Check sheet for the modelled part. Datum: model origin and axes. Units: mm. A direction names the side the tool comes from. Give positions to 0.01 mm unless a question says otherwise; leave off trailing zeros. Write each loop counter-clockwise with the first axis right and the second up, starting at its lowest first coordinate (ties: lowest second). Pieces come first, ordered by that corner, then holes.
from build123d import *

# Parameters (mm, degrees)
SKETCH1_W           = 90
SKETCH1_H           = 45
BOSS_EXTRUDE1_DEPTH = 117
SKETCH1_3_W         = 90
SKETCH1_3_H         = 36
BOSS_EXTRUDE2_DEPTH = 45
BOSS_EXTRUDE3_DEPTH = 27
RIB2_REACH          = 188.435
SKETCH2_WALL_W      = 425.781638764
SKETCH2_WALL_H      = 18
CUT_EXTRUDE1_REACH  = 158.087
SKETCH3_R           = 27


with BuildPart() as part:
    # Sketch1 → Boss-Extrude1 (new body)
    with BuildSketch(Plane.XY):
        with Locations((0, 22.5)):
            Rectangle(SKETCH1_W, SKETCH1_H)
    extrude(amount=BOSS_EXTRUDE1_DEPTH)

    # Sketch1_3 → Boss-Extrude2 (add)
    with BuildSketch(Plane.XY):
        with Locations((0, 63)):
            Rectangle(SKETCH1_3_W, SKETCH1_3_H)
    extrude(amount=BOSS_EXTRUDE2_DEPTH)

    # Sketch1_4 → Boss-Extrude3 (add)
    with BuildSketch(Plane.XY):
        with BuildLine():
            ThreePointArc((-45, 93), (0, 138), (45, 93))
            Line((45, 93), (45, 81))
            Line((45, 81), (-45, 81))
            Line((-45, 81), (-45, 93))
        make_face()
        with BuildLine():
            Line((-27, 93), (27, 93))
            ThreePointArc((27, 93), (0, 120), (-27, 93))
        make_face(mode=Mode.SUBTRACT)
    extrude(amount=BOSS_EXTRUDE3_DEPTH)

    # Sketch2 wall → Rib2 (add, up to next)
    with BuildSketch(Plane(origin=(0, 63, 63), x_dir=(0, -0.707106781187, 0.707106781187), z_dir=(0, -0.707106781187, -0.707106781187)), mode=Mode.PRIVATE) as rib2_sk1:
        Rectangle(SKETCH2_WALL_W, SKETCH2_WALL_H)
    rib2_tool1 = extrude(rib2_sk1.sketch, amount=RIB2_REACH, mode=Mode.PRIVATE) - part.part
    add(rib2_tool1.solids().sort_by_distance((0, 63, 63))[0])

    # Sketch3 → Cut-Extrude1 (cut, up to next)
    with BuildSketch(Plane(origin=(0, 45, 0), x_dir=(1, 0, 0), z_dir=(0, 1, 0)), mode=Mode.PRIVATE) as cut_extrude1_sk1:
        with Locations((0, -117)):
            Circle(SKETCH3_R)
    cut_extrude1_tool1 = extrude(cut_extrude1_sk1.sketch, amount=-CUT_EXTRUDE1_REACH, mode=Mode.PRIVATE) & part.part
    add(cut_extrude1_tool1.solids().sort_by_distance((0, 45, 117))[0], mode=Mode.SUBTRACT)


solid = part.part
1) Gauge pin test, flat ends, axial feed: pin 1 (5 mm diameter, centred on x = -28, y = 99.5, fed in from +Z); pin 2 (11 mm diameter, centred on x = -20, y = 70, fed in from +Z); pin 3 (11 mm diameter, centred on y = 59, z = 71.5, fed in from -X); pin 4 (1 mm diameter, centred on x = -12.5, y = 14, fed in from -Z). Record the tip position at first contact, or that the pin passes through.
2) Sectioned sample at C-C on z = 63. Record the boundary of the cut face in (x, y), then the cut area to 3 significant figures.
3) Access from +Z, -Z, +X, -X, +Y, -Y to the whole of each face (thin tool, end or side, straight path). Record for faces 4 (the flat face through (9, 56, 56)), 5 (the flat face through (1, 91, 27)), 6 (the flat face through (9.4, 45, 80.5)), 7 (the flat face through (0, 93, 13)), 8 (the flat face through (-27, 63, 45)).
4) Sectioned sample at A-A on x = 0. Record the boundary of the cut face in (y, z), then the cut area to 3 significant figures.
5) Sectioned sample at B-B on y = 33.5. Record the boundary of the cut face in (x, z), then the cut area to 3 significant figures.
6) Scan lines: L1, parallel to Y at x = -0.5, z = 23.5; L2, parallel to Y at x = 34, z = 110. Record each from-to range of solid material in increasing order.
7) Sectioned sample at D-D on y = 109. Record the boundary of the cut face in (x, z).
8) Draft check along Y on faces 1 (the flat face through (-36, 23, 117)), 2 (the flat face through (-1, 0, 58)), 3 (the cylindrical face through (0.594, 119.993, 13.311)). Enter one of: +Y half, -Y half, draft (parallel to the pull), parting line (faces both ways), or undercut.
Answers below:
1. pin 1: stops at z = 27
1. pin 2: stops at z = 45
1. pin 3: stops at x = -9
1. pin 4: stops at z = 0
2. outline: (-45, 0) - (45, 0) - (45, 45) - (9, 45) - (9, 63) - (-9, 63) - (-9, 45) - (-45, 45) - close
2. area: 4,370 mm2
3. face 4: +Z, +X, +Y
3. face 5: +Z, +X, -X, +Y
3. face 6: +Z, +Y
3. face 7: +Z, -Z
3. face 8: +Z, -X, +Y
4. outline: (0, 0) - (93, 0) - (93, 27) - (81, 27) - (81, 45) - (45, 81) - (45, 90) - (0, 90) - close; (120, 0) - (138, 0) - (138, 27) - (120, 27) - close
4. area: 7,130 mm2
5. outline: (-45, 0) - (45, 0) - (45, 117) - (27, 117) arc R27 cw to (-27, 117) - (-45, 117) - close
5. area: 9,380 mm2
6. L1: y = 0 to 93, 120 to 138
6. L2: y = 0 to 45
7. outline: (-42.06, 0) - (-21.75, 0) - (-21.75, 27) - (-42.06, 27) - close; (21.75, 0) - (42.06, 0) - (42.06, 27) - (21.75, 27) - close
8. face 1: draft
8. face 2: -Y half
8. face 3: undercut
